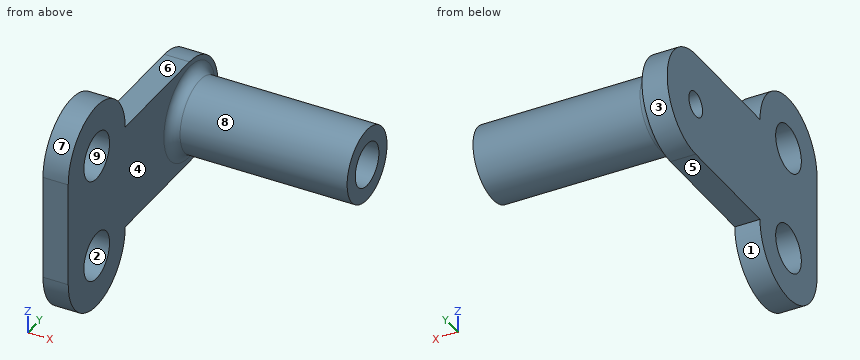
```python
from build123d import *

# Parameters (mm, degrees)
SKETCH_1_R      = 2.25
SKETCH_1_R_2    = 2.075
EXTRUDE_1_DEPTH = 2.4
SKETCH_4_R      = 3.5
SKETCH_4_R_2    = 2.075
EXTRUDE_2_DEPTH = 16.9
FILLET_1_R      = 1
SKETCH_5_R      = 2.075
SKETCH_5_R_2    = 1.2
EXTRUDE_3_DEPTH = 4


with BuildPart() as part:
    # 草图1 → 凸台-拉伸1 (new body)
    with BuildSketch(Plane(origin=(0, 0, 0), x_dir=(0, 0, -1), z_dir=(1, 0, 0))):
        with BuildLine():
            Line((-5, 0), (5, 0))
            ThreePointArc((5, 0), (10, 5), (5, 10))
            Line((5, 10), (5, 21.282156306))
            ThreePointArc((5, 21.282156306), (0, 26.282156306), (-5, 21.282156306))
            Line((-5, 21.282156306), (-5, 10))
            ThreePointArc((-5, 10), (-10, 5), (-5, 0))
        make_face()
        with Locations((-5, 5)):
            Circle(SKETCH_1_R, mode=Mode.SUBTRACT)
        with Locations((5, 5)):
            Circle(SKETCH_1_R, mode=Mode.SUBTRACT)
        with Locations((0, 21.282156306)):
            Circle(SKETCH_1_R_2, mode=Mode.SUBTRACT)
    extrude(amount=EXTRUDE_1_DEPTH)

    # 草图4 → 凸台-拉伸2 (add)
    with BuildSketch(Plane(origin=(2.4, 0, 0), x_dir=(0, 0, -1), z_dir=(1, 0, 0))):
        with Locations((0, 21.282156306)):
            Circle(SKETCH_4_R)
        with Locations((0, 21.282156306)):
            Circle(SKETCH_4_R_2, mode=Mode.SUBTRACT)
    extrude(amount=EXTRUDE_2_DEPTH)

    # 圆角1
    fillet_1_edges = [part.edges().sort_by_distance(p)[0] for p in [
        (2.4, 21.282156306, 3.5),
    ]]
    fillet(fillet_1_edges, radius=FILLET_1_R)

    # 草图5 → 凸台-拉伸3 (add)
    with BuildSketch(Plane.ZY):
        with Locations((0, 21.282156306)):
            Circle(SKETCH_5_R)
        with Locations((0, 21.282156306)):
            Circle(SKETCH_5_R_2, mode=Mode.SUBTRACT)
    extrude(amount=-EXTRUDE_3_DEPTH)


solid = part.part
```
Design review of the part built by this model. Coordinates are the model's own, in mm. Face numbers are marked on the shaded views. A direction names the side the tool comes from. Round coordinates to 2 decimals unless told otherwise and drop trailing zeros. Write each loop counter-clockwise with the first axis right and the second up, starting at its lowest first coordinate (ties: lowest second). Pieces come first, ordered by that corner, then holes. Notation, with made-up numbers: (-13, 48) -> (-8, 48) arc R19 ccw to (-8, 58) -> close; hole circle Ø1 at (26, 36). An arc over 180 degrees is marked (long way). Write item = value, one per line. Start each with the question number.
1) Take a section at D-D, the plane y = 15. State the section outline as (x, z) points.
2) Take a section at A-A, the plane z = 0. State the section outline as (x, y) points.
3) Tool access review of the marked faces 5, 6, 7, 8 and 9: name each direction out of +Z, -Z, +X, -X, +Y, -Y from which nothing blocks a thin tool from reaching the whole face with its end or side.
4) Mouldability with a two-part tool opening along Z and no side actions: class the marked faces 1, 2, 3 and 4 as +Z half, -Z half, draft (parallel to the pull), parting line (faces both ways), or undercut.
5) Clearance check with flat-ended pins moving along their axes: pin 1 (2.5 mm diameter, centred on x = 1, y = 14, fed in from +Z); pin 2 (5 mm diameter, centred on x = 6, z = 6.5, fed in from +Y); pin 3 (1 mm diameter, centred on x = 13, y = 20, fed in from -Z); pin 4 (2.5 mm diameter, centred on x = 1.5, y = 15.5, fed in from -Z). State where each tip first meets the part, or that it passes through.
6) Take a section at C-C, the plane x = 17. State the section outline as (y, z) points (3 decimals).
7) Take a section at B-B, the plane y = 5. State the section outline as (x, z) points.
8) Wall thickness on probe 1 along Y at (x, z) = (15.75, 0); probe 2 along Y at (x, z) = (1.6, 0); probe 3 along X at (y, z) = (10.75, 2): over which ranges is each line inside the solid? List them lowest first. Write a range as from..to.
Results list:
q1.outline = (0, -5) -> (2.4, -5) -> (2.4, 5) -> (0, 5) -> close
q2.outline = (0, 0) -> (2.4, 0) -> (2.4, 16.78) arc R1 cw to (3.4, 17.78) -> (19.3, 17.78) -> (19.3, 19.21) -> (4, 19.21) -> (4, 20.08) -> (0, 20.08) -> close; (0, 22.48) -> (4, 22.48) -> (4, 23.36) -> (19.3, 23.36) -> (19.3, 24.78) -> (3.4, 24.78) arc R1 cw to (2.4, 25.78) -> (2.4, 26.28) -> (0, 26.28) -> close
q3.face_5 = -Z, +X, -X, +Y
q3.face_6 = +Z, +X, -X, +Y
q3.face_7 = +Z, +X, -X
q3.face_8 = +X
q3.face_9 = +X, -X
q4.face_1 = -Z half
q4.face_2 = undercut
q4.face_3 = parting line
q4.face_4 = draft
q5.pin_1 = 5
q5.pin_2 = through
q5.pin_3 = -3.41
q5.pin_4 = -5
q6.outline = circle Ø7 at (21.282, 0); hole circle Ø4.15 at (21.282, 0)
q7.outline = (0, -10) -> (2.4, -10) -> (2.4, -7.25) -> (0, -7.25) -> close; (0, -2.75) -> (2.4, -2.75) -> (2.4, 2.75) -> (0, 2.75) -> close; (0, 7.25) -> (2.4, 7.25) -> (2.4, 10) -> (0, 10) -> close
q8.probe_1 = 17.78..19.21, 23.36..24.78
q8.probe_2 = 0..20.08, 22.48..26.28
q8.probe_3 = 0..2.4
